Part model, mm, in its own coordinate system. A direction names the side the tool comes from. Give positions to 0.01 mm unless a question says otherwise; leave off trailing zeros. Order: outer loops, then holes, each group sorted by start corner. A loop starts at its lowest first (then second) coordinate and runs counter-clockwise, first axis right, second up. Notation, with made-up numbers: M 35.5,3.5 L 83.5,3.5 A30 cw 83.5,26.5 Z; hole C 32.25,51 d4. An arc over 180 degrees is marked long. One line per question, with ' | ' between items.
```python
from build123d import *

# Parameters (mm, degrees)
SKETCH_R        = 33
PAD_DEPTH       = 26
POCKET_DEPTH    = 12
SKETCH002_R     = 23
SKETCH002_R_2   = 8
POCKET001_DEPTH = 12
SKETCH003_R     = 8
POCKET002_DEPTH = 2
CHAMFER_SIZE    = 1.6


with BuildPart() as part:
    # Sketch → Pad (new body)
    with BuildSketch(Plane.XY):
        Circle(SKETCH_R)
    extrude(amount=PAD_DEPTH)

    # Sketch001 → Pocket (cut)
    with BuildSketch(Plane.XY):
        with BuildLine():
            ThreePointArc((-1.5, -2.598076), (3, 0), (-1.5, 2.598076))
            Line((-1.5, 2.598076), (-1.5, -2.598076))
        make_face()
    extrude(amount=POCKET_DEPTH, mode=Mode.SUBTRACT)

    # Sketch002 (on Face2 of Pad) → Pocket001 (cut)
    with BuildSketch(Plane(origin=(0, 0, 0), x_dir=(1, 0, 0), z_dir=(0, 0, -1))):
        Circle(SKETCH002_R)
        Circle(SKETCH002_R_2, mode=Mode.SUBTRACT)
    extrude(amount=-POCKET001_DEPTH, mode=Mode.SUBTRACT)

    # Sketch003 (on Face7 of Pocket001) → Pocket002 (cut)
    with BuildSketch(Plane(origin=(0, 0, 0), x_dir=(1, 0, 0), z_dir=(0, 0, -1))):
        Circle(SKETCH003_R)
    extrude(amount=-POCKET002_DEPTH, mode=Mode.SUBTRACT)

    # Chamfer
    chamfer_edges = [part.edges().sort_by_distance(p)[0] for p in [
        (-33, 0, 26),
    ]]
    chamfer(chamfer_edges, length=CHAMFER_SIZE)


with BuildPart() as part_1:
    # Body placement: moved
    add(part.part.moved(Location((0, 0, 1.4))))


solid = part_1.part
```
1. Slice it at D-D on z = 19. Give the cut face in (x, y), then the cut area to 3 significant figures.
Worked out:
outline: C 0,0 d66 | area: 3,420 mm2
2. Probe L1, parallel to Y at x = 0, z = 7.25; L2, parallel to Y at x = 5, z = 7.5 (3 decimals); L3, parallel to X at y = -20, z = 7.25. List the from-to ranges inside material, lowest first. Write a range as from..to.
Worked out:
L1: y = -33..-23, -8..-3, 3..8, 23..33 | L2: y = -32.619..-22.45, -6.245..6.245, 22.45..32.619 | L3: x = -26.25..-11.36, 11.36..26.25
3. Drop flat-ended pins along their axis: pin 1 (14 mm diameter, centred on x = -2.5, y = -10.5, fed in from -Z); pin 2 (12 mm diameter, centred on x = -17, z = 24, fed in from -Y); pin 3 (6 mm diameter, centred on y = 6, z = 24, fed in from -X). Give the stop position or say it passes through.
Worked out:
pin 1: stops at z = 3.4 | pin 2: stops at y = -31.11 | pin 3: stops at x = -32.86
4. Slice it at C-C on x = 0. Give the cut face in (y, z).
Worked out:
outline: M -33,1.4 L -23,1.4 L -23,13.4 L -8,13.4 L -8,3.4 L -3,3.4 L -3,13.4 L 3,13.4 L 3,3.4 L 8,3.4 L 8,13.4 L 23,13.4 L 23,1.4 L 33,1.4 L 33,25.8 L 31.4,27.4 L -31.4,27.4 L -33,25.8 Z
5. Slice it at B-B on y = 0. Give the cut face in (x, z).
Worked out:
outline: M -33,1.4 L -23,1.4 L -23,13.4 L -8,13.4 L -8,3.4 L -1.5,3.4 L -1.5,13.4 L 3,13.4 L 3,3.4 L 8,3.4 L 8,13.4 L 23,13.4 L 23,1.4 L 33,1.4 L 33,25.8 L 31.4,27.4 L -31.4,27.4 L -33,25.8 Z
6. Slice it at A-A on z = 7. Give the cut face in (x, y), then the cut area to 3 significant figures.
Worked out:
outline: C 0,0 d66; C 0,0 d16; hole C 0,0 d46; hole M -1.5,-2.6 A3 ccw long -1.5,2.6 Z | area: 1,940 mm2
7. Mould opens along X. For faces 1 (the flat face through (6.9, 22.5, 1.4)), 2 (the flat face through (10, 0, 13.4)), 3 (the cylindrical face through (30.5, -12.6, 13.4)) say: released by +X, released by -X, zero draft, split by the parting line, or undercut.
Worked out:
face 1: zero draft | face 2: undercut | face 3: split by the parting line
8. Tool access for faces 4 (the flat face through (0, 0, 27.4)), 5 (the flat face through (0, 0, 13.4)): list every direction of +Z, -Z, +X, -X, +Y, -Y with a clear straight run to the whole face (end or side of a thin tool).
Worked out:
face 4: +Z, +X, -X, +Y, -Y | face 5: -Z
